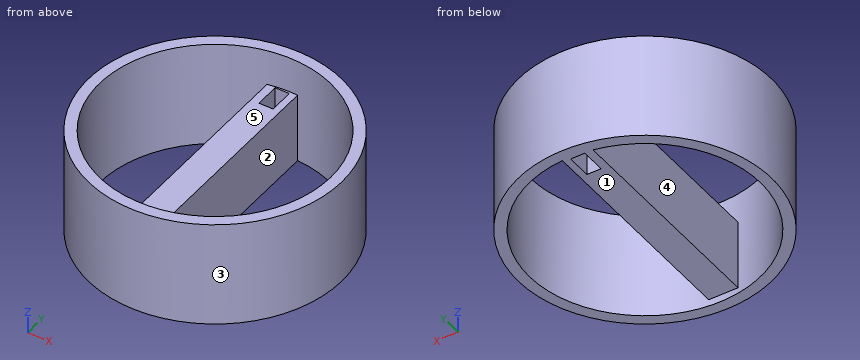
```python
from build123d import *

# Parameters (mm, degrees)
F0_R     = 35.715838
F1_DEPTH = 30
F2_R     = 32.580129
F3_DEPTH = 149
F5_DEPTH = 19.8
F6_W     = 4.003989
F6_H     = 7.003708
F7_DEPTH = 120.5


with BuildPart() as f1:
    # F0 (on Top) → F1 (new body)
    with BuildSketch(Plane.XY):
        Circle(F0_R)
    extrude(amount=F1_DEPTH)

    # F2 (on face) → F3 (cut)
    with BuildSketch(Plane(origin=(0, 0, 0), x_dir=(1, 0, 0), z_dir=(0, 0, -1))):
        Circle(F2_R)
    extrude(amount=-F3_DEPTH, mode=Mode.SUBTRACT)

    # F4 (on Top) → F5 (join)
    with BuildSketch(Plane.XY):
        Polygon((1.966494, 35.009865), (-6.307223, 34.134421), (-6.307223, -30.437076), (1.966494, -30.437076), align=None)
    extrude(amount=F5_DEPTH)

    # F6 (on face) → F7 (cut)
    with BuildSketch(Plane.XY.offset(19.8)):
        with Locations((-2.001994, 28.461934)):
            Rectangle(F6_W, F6_H)
    extrude(amount=-F7_DEPTH, mode=Mode.SUBTRACT)


solid = f1.part
```
The listing builds one solid part. Answer for the finished solid, in the listing's coordinates (mm). Face numbers are marked on the shaded views. A direction names the side the tool comes from. Coordinates: 2 decimals unless noted, no trailing zeros. Write each loop counter-clockwise with the first axis right and the second up, starting at its lowest first coordinate (ties: lowest second). Pieces come first, ordered by that corner, then holes.
Q1. Section C-C, the plane x = -25 is taken. Write down the section's boundary in (y, z), then the cut area to 3 significant figures.
Returned:
outline: (-25.51, 0) - (-20.89, 0) - (-20.89, 30) - (-25.51, 30) - close; (20.89, 0) - (25.51, 0) - (25.51, 30) - (20.89, 30) - close
area: 277 mm2
Q2. Section B-B, the plane z = 13.5 is taken. Write down the section's boundary in (x, y), then the cut area to 3 significant figures.
Returned:
outline: circle Ø71.43 at (0, 0); hole (-6.31, -30.44) - (-6.31, 31.96) arc R32.58 ccw (long way) to (1.97, 32.52) - (1.97, -30.44) - close; hole (-4, 24.96) - (0, 24.96) - (0, 31.96) - (-4, 31.96) - close
area: 1,160 mm2
Q3. The mould has two halves that part along X. Classify the marked faces 1, 2 and 3: released by +X, released by -X, zero draft, split by the parting line, or undercut.
Returned:
face 1: zero draft
face 2: undercut
face 3: split by the parting line
Q4. Find the intervals of material crossed by line 1 along Y through (x, z) = (0, 21.5); line 2 along X through (y, z) = (27, 14.5); line 3 along Y through (x, z) = (21, 19), in increasing order.
Returned:
line 1: y = -35.72 to -32.58, 32.58 to 35.72
line 2: x = -23.38 to -18.23, -6.31 to -4, 0 to 1.97, 18.23 to 23.38
line 3: y = -28.89 to -24.91, 24.91 to 28.89
Q5. Which of the six approach directions +Z, -Z, +X, -X, +Y, -Y give full straight-line access (tool end or side, diameter ignored) to the marked faces 4 and 5?
Returned:
face 4: +Z, -Z
face 5: +Z
Q6. Section A-A, the plane y = 0 is taken. Write down the section's boundary in (x, z).
Returned:
outline: (-35.72, 0) - (-32.58, 0) - (-32.58, 30) - (-35.72, 30) - close; (-6.31, 0) - (1.97, 0) - (1.97, 19.8) - (-6.31, 19.8) - close; (32.58, 0) - (35.72, 0) - (35.72, 30) - (32.58, 30) - close
Q7. Section D-D, the plane x = -1 is taken. Write down the section's boundary in (y, z).
Returned:
outline: (-35.7, 0) - (-32.56, 0) - (-32.56, 30) - (-35.7, 30) - close; (-30.44, 0) - (24.96, 0) - (24.96, 19.8) - (-30.44, 19.8) - close; (31.96, 0) - (35.7, 0) - (35.7, 30) - (32.56, 30) - (32.56, 19.8) - (31.96, 19.8) - close
Q8. Given P1, Ø7.5, axis at y = 28, z = 9, coming from the +X side; P2, Ø3, axis at x = 25, z = 13.5, coming from the +Y side; P3, Ø4, axis at x = -3.5, z = 13.5, coming from the -Y side, each flat-ended and moving along its own axis, determine where each tip first touches the part or whether it passes through.
Returned:
P1: stops at x = 26.22
P2: stops at y = 26.9
P3: stops at y = -35.68
